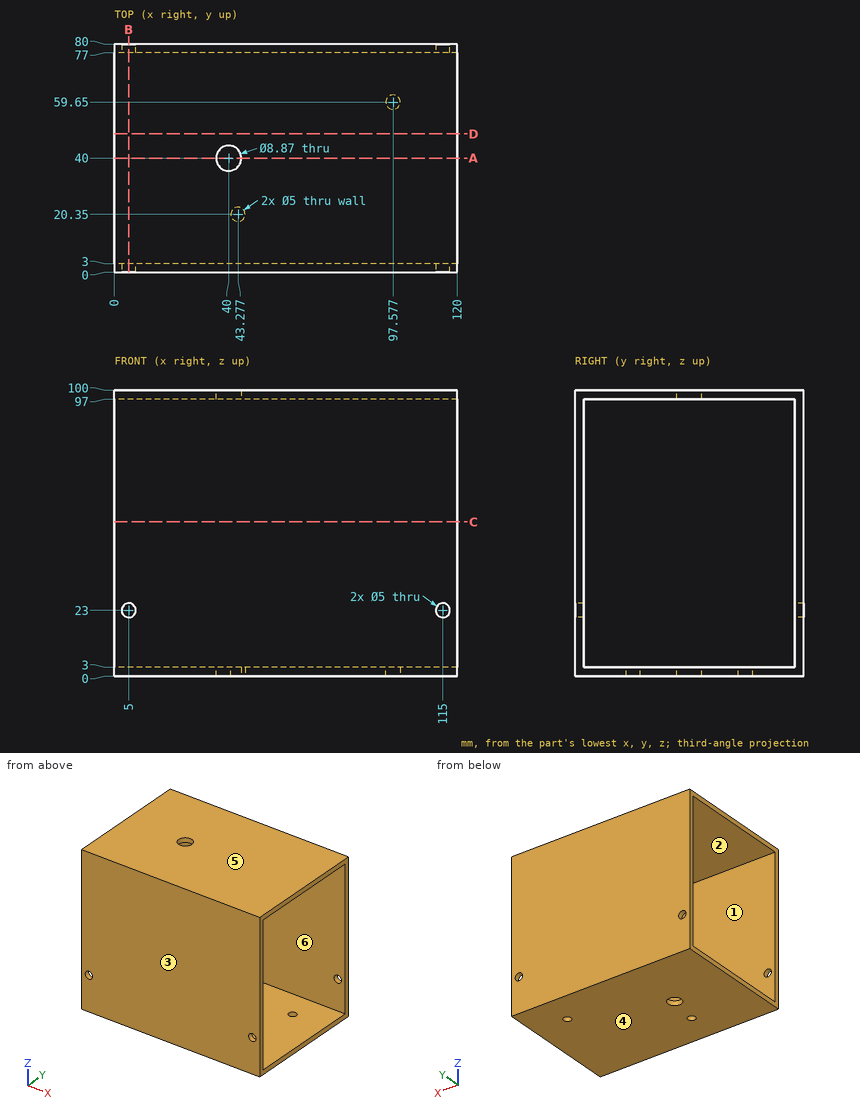
Check sheet for the drawn part. Datum: minimum x, y, z corner. Units: mm. A direction names the side the tool comes from. Round coordinates to 2 decimals unless told otherwise and drop trailing zeros. Order: outer loops, then holes, each group sorted by start corner. A loop starts at its lowest first (then second) coordinate and runs counter-clockwise, first axis right, second up. Notation, with made-up numbers: (-19, 17.25) -> (12, 17.25) arc R28 cw to (12, 38.25) -> close; hole circle Ø5 at (57, 1). An arc over 180 degrees is marked (long way). Put each result on its own line as item: value. Start each with the question number.
(1) Draft check along Y on the marked faces 1, 2, 3 and 4. Enter one of: +Y half, -Y half, draft (parallel to the pull), parting line (faces both ways), or undercut.
(2) Section check A-A (y = 40). Enter the section's corners in (x, z) (3 decimals).
(3) Material ranges on line 1 along Z through (x, y) = (101.5, 35); line 2 along Y through (x, z) = (104.5, 92); line 3 along Z through (x, y) = (115, 1), recorded low to high.
(4) Section check C-C (z = 54). Enter the section's corners in (x, y).
(5) Tool access check on the marked faces 5 and 6. Record the directions out of +Z, -Z, +X, -X, +Y, -Y that give a thin tool (end or side, any length) a straight path to the whole face; none if there is none.
(6) Depth check by flat-ended pin: pin 1 Ø4 at (x, z) = (5, 23) entering from +Y. Enter the tip coordinate at first touch or a pass-through.
(7) Section check B-B (x = 5). Enter the section's corners in (y, z).
(8) Section check D-D (y = 48.5). Enter the section's corners in (x, z).
Completed:
1. face 1: undercut
1. face 2: undercut
1. face 3: -Y half
1. face 4: draft
2. outline: (0, 0) -> (35.565, 0) -> (35.565, 3) -> (0, 3) -> close; (0, 97) -> (35.565, 97) -> (35.565, 100) -> (0, 100) -> close; (44.435, 0) -> (120, 0) -> (120, 3) -> (44.435, 3) -> close; (44.435, 97) -> (120, 97) -> (120, 100) -> (44.435, 100) -> close
3. line 1: z = 0 to 3, 97 to 100
3. line 2: y = 0 to 3, 77 to 80
3. line 3: z = 0 to 20.5, 25.5 to 100
4. outline: (0, 0) -> (120, 0) -> (120, 3) -> (0, 3) -> close; (0, 77) -> (120, 77) -> (120, 80) -> (0, 80) -> close
5. face 5: +Z, +X, -X, +Y, -Y
5. face 6: +X, -X
6. pin 1: passes through
7. outline: (0, 0) -> (80, 0) -> (80, 20.5) -> (77, 20.5) -> (77, 3) -> (3, 3) -> (3, 20.5) -> (0, 20.5) -> close; (0, 25.5) -> (3, 25.5) -> (3, 97) -> (77, 97) -> (77, 25.5) -> (80, 25.5) -> (80, 100) -> (0, 100) -> close
8. outline: (0, 0) -> (120, 0) -> (120, 3) -> (0, 3) -> close; (0, 97) -> (120, 97) -> (120, 100) -> (0, 100) -> close
